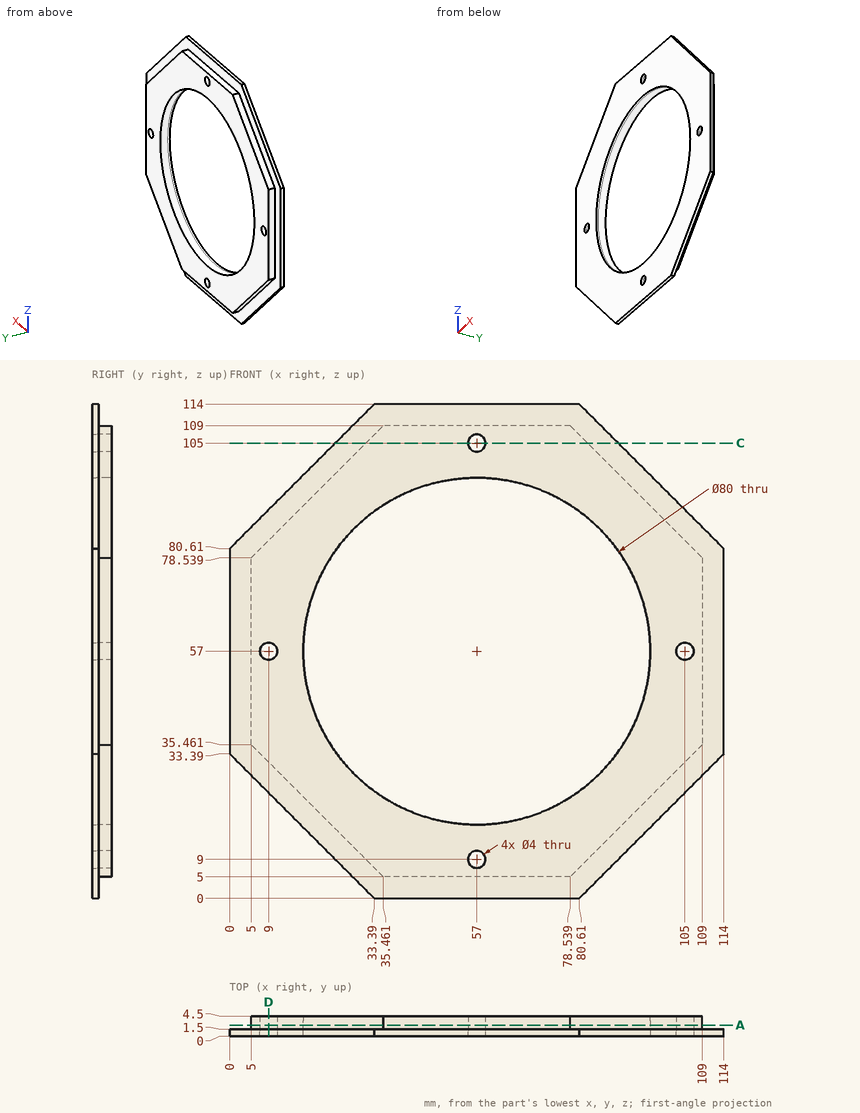
Geometry check sheet. Reference: drawing and pictorial views, mm from the part's lowest x, y, z. Give positions to 0.01 mm unless a question says otherwise; leave off trailing zeros. Loops run counter-clockwise (first coordinate to the right, second up) from the corner with the lowest first, then second, coordinate; pieces in that order, holes last. Notation, with made-up numbers: (48.5, 41.5) - (101.5, 41.5) arc R27 ccw to (101.5, 79.5) - close; hole circle Ø2 at (-39, 63.5). An arc over 180 degrees is marked (long way). One line per question, with ' | ' between items. Start each with the question number.
1. Cross-section at D-D, the plane x = 9. Enter the section's corners in (y, z).
2. Material ranges on line 1 along Z through (x, y) = (57, 0.4); line 2 along Z through (x, y) = (69.5, 4.3); line 3 along X through (y, z) = (2.3, 60.5), recorded low to high. Write a range as [from, to].
3. Cross-section at C-C, the plane z = 105. Enter the section's corners in (x, y).
4. Cross-section at A-A, the plane y = 2.5. Enter the section's corners in (x, z), plus the area to 3 significant figures.
5. Gauge pin test, flat ends, axial feed: pin 1 Ø2.5 at (y, z) = (3, 49.5) entering from -X; pin 2 Ø0.9 at (x, y) = (59.5, 3) entering from -Z; pin 3 Ø0.9 at (x, y) = (52, 3) entering from +Z; pin 4 Ø3.5 at (x, z) = (57, 9) entering from -Y. Record the tip position at first contact, or that the pin passes through.
Check result:
1) outline: (0, 24.39) - (1.5, 24.39) - (1.5, 31.46) - (4.5, 31.46) - (4.5, 55) - (0, 55) - close; (0, 59) - (4.5, 59) - (4.5, 82.54) - (1.5, 82.54) - (1.5, 89.61) - (0, 89.61) - close
2) line 1: z = [0, 7], [11, 17], [97, 103], [107, 114] | line 2: z = [5, 19], [95, 109] | line 3: x = [5, 17.15], [96.85, 109]
3) outline: (24.39, 0) - (55, 0) - (55, 4.5) - (31.46, 4.5) - (31.46, 1.5) - (24.39, 1.5) - close; (59, 0) - (89.61, 0) - (89.61, 1.5) - (82.54, 1.5) - (82.54, 4.5) - (59, 4.5) - close
4) outline: (5, 35.46) - (35.46, 5) - (78.54, 5) - (109, 35.46) - (109, 78.54) - (78.54, 109) - (35.46, 109) - (5, 78.54) - close; hole circle Ø4 at (9, 57); hole circle Ø80 at (57, 57); hole circle Ø4 at (57, 9); hole circle Ø4 at (57, 105); hole circle Ø4 at (105, 57) | area: 3,880 mm2
5) pin 1: stops at x = 5 | pin 2: stops at z = 5 | pin 3: stops at z = 109 | pin 4: passes through
